Source: CAD feature listing. Evaluate the final solid. Frame: model axes, mm. Round coordinates to 2 decimals unless told otherwise and drop trailing zeros. Loops run counter-clockwise (first coordinate to the right, second up) from the corner with the lowest first, then second, coordinate; pieces in that order, holes last. Notation, with made-up numbers: M -20,49 L 6,49 A9 cw 6,63 Z; hole C 62.5,-25 d2. An arc over 180 degrees is marked long. Write each question's results on one line, items separated by ' | '. Start each with the question number.
1. Ray query, line 1 (X direction, y = 2.2, z = 9.5); line 2 (Z direction, x = 26, y = 3); line 3 (X direction, y = 5.25, z = 8.5). Return the intervals inside material, ascending.
2. Section D-D on z = 0. Output: boundary loops of the cut face in (x, y).
3. Section C-C on y = 4. Output: boundary loops of the cut face in (x, z).
4. Section A-A on z = 9.5. Output: boundary loops of the cut face in (x, y).
5. Draft query along Z for faces 1 (the flat face through (0, 5.78, 0)), 2 (the cylindrical face through (-26.35, 2.85, -7.94)), 3 (the cylindrical face through (-8.806, 8.787, -2.643)). Return one class per face: released by +Z, released by -Z, zero draft, split by the parting line, or undercut.
6. Section B-B on x = 26. Output: boundary loops of the cut face in (y, z), and give its area (3 significant figures).
7. Contact query for a flat-ended pin moving along its axis: pin 1 Ø4 at (x, z) = (-26, -9.5) entering from +Y. Output: stop coordinate, or through.
from build123d import *

# Parameters (mm, degrees)
SKETCH2_R           = 1.6
BOSS_EXTRUDE1_DEPTH = 5.78
SKETCH3_R           = 8.8
BOSS_EXTRUDE2_DEPTH = 6.1


with BuildPart() as part:
    # Sketch2 → Boss-Extrude1 (new body)
    with BuildSketch(Plane(origin=(0, 0, 0), x_dir=(1, 0, 0), z_dir=(0, 1, 0))):
        with BuildLine():
            Line((-26.8, -13.5), (26.8, -13.5))
            ThreePointArc((26.8, -13.5), (29.0627417, -12.5627417), (30, -10.3))
            Line((30, -10.3), (30, 10.3))
            ThreePointArc((30, 10.3), (29.0627417, 12.5627417), (26.8, 13.5))
            Line((26.8, 13.5), (-26.8, 13.5))
            ThreePointArc((-26.8, 13.5), (-29.0627417, 12.5627417), (-30, 10.3))
            Line((-30, 10.3), (-30, -10.3))
            ThreePointArc((-30, -10.3), (-29.0627417, -12.5627417), (-26.8, -13.5))
        make_face()
        with Locations((26, 9.5)):
            Circle(SKETCH2_R, mode=Mode.SUBTRACT)
        with Locations((-26, 9.5)):
            Circle(SKETCH2_R, mode=Mode.SUBTRACT)
        with Locations((-26, -9.5)):
            Circle(SKETCH2_R, mode=Mode.SUBTRACT)
        with Locations((26, -9.5)):
            Circle(SKETCH2_R, mode=Mode.SUBTRACT)
    extrude(amount=BOSS_EXTRUDE1_DEPTH)

    # Sketch3 → Boss-Extrude2 (add)
    with BuildSketch(Plane(origin=(0, 5.78, 0), x_dir=(1, 0, 0), z_dir=(0, 1, 0))):
        with Locations((-17.2, 0)):
            Circle(SKETCH3_R)
    extrude(amount=BOSS_EXTRUDE2_DEPTH)


solid = part.part
Taken from the geometry:
1) line 1: -30 to -27.6, -24.4 to 24.4, 27.6 to 30 | line 2: -13.5 to -11.1, -7.9 to 7.9, 11.1 to 13.5 | line 3: -30 to -27.25, -24.75 to 24.75, 27.25 to 30
2) outline: M -30,0 L 30,0 L 30,5.78 L -8.4,5.78 L -8.4,11.88 L -26,11.88 L -26,5.78 L -30,5.78 Z
3) outline: M -30,-10.3 A3.2 ccw -26.8,-13.5 L 26.8,-13.5 A3.2 ccw 30,-10.3 L 30,10.3 A3.2 ccw 26.8,13.5 L -26.8,13.5 A3.2 ccw -30,10.3 Z; hole C -26,-9.5 d3.2; hole C -26,9.5 d3.2; hole C 26,-9.5 d3.2; hole C 26,9.5 d3.2
4) outline: M -30,0 L -27.6,0 L -27.6,5.78 L -30,5.78 Z; M -24.4,0 L 24.4,0 L 24.4,5.78 L -24.4,5.78 Z; M 27.6,0 L 30,0 L 30,5.78 L 27.6,5.78 Z
5) face 1: zero draft | face 2: undercut | face 3: split by the parting line
6) outline: M 0,-13.5 L 5.78,-13.5 L 5.78,-11.1 L 0,-11.1 Z; M 0,-7.9 L 5.78,-7.9 L 5.78,7.9 L 0,7.9 Z; M 0,11.1 L 5.78,11.1 L 5.78,13.5 L 0,13.5 Z | area: 119 mm^2
7) pin 1: y = 5.78
